from build123d import *

# Parameters (mm, degrees)
SKETCH1_R           = 2
BOSS_EXTRUDE1_DEPTH = 25
BOSS_EXTRUDE2_START = -25
SKETCH3_R           = 7
SKETCH3_R_2         = 2
BOSS_EXTRUDE2_DEPTH = 25
MOVE_FACE1_BY       = 2
MOVE_FACE1_2_BY     = 2
BOSS_EXTRUDE3_START = -25
BOSS_EXTRUDE3_DEPTH = 25


with BuildPart() as part:
    # Sketch1 → Boss-Extrude1 (new body)
    with BuildSketch(Plane(origin=(0, 0, 0), x_dir=(1, 0, 0), z_dir=(0, 1, 0))):
        with BuildLine():
            Line((-5, 0), (-5, 29.5))
            ThreePointArc((-5, 29.5), (0, 34.5), (5, 29.5))
            Line((5, 29.5), (5, 0))
            ThreePointArc((5, 0), (0, -5), (-5, 0))
        make_face()
        with Locations(Location((0, 29.5, 0), (0, 0, 270))):
            Circle(SKETCH1_R, mode=Mode.SUBTRACT)
        with Locations(Location((0, 0, 0), (0, 0, 270))):
            Circle(SKETCH1_R, mode=Mode.SUBTRACT)
    extrude(amount=BOSS_EXTRUDE1_DEPTH)

    # Sketch3 → Boss-Extrude2 (add)
    # profile 1 of 2: a face of its own
    with BuildSketch(Plane(origin=(0, 25, 0), x_dir=(1, 0, 0), z_dir=(0, 1, 0)).offset(BOSS_EXTRUDE2_START)):
        with Locations((0, 29.5)):
            Circle(SKETCH3_R)
        with Locations(Location((0, 29.5, 0), (0, 0, 270))):
            Circle(SKETCH3_R_2, mode=Mode.SUBTRACT)
    # profile 2 of 2: a face of its own
    with BuildSketch(Plane(origin=(0, 25, 0), x_dir=(1, 0, 0), z_dir=(0, 1, 0)).offset(BOSS_EXTRUDE2_START)):
        Circle(SKETCH3_R)
        with Locations(Location((0, 0, 0), (0, 0, 270))):
            Circle(SKETCH3_R_2, mode=Mode.SUBTRACT)
    extrude(amount=BOSS_EXTRUDE2_DEPTH)

    # Move Face1: a curved face moved inward by 2.0
    add(Solid.thicken(part.faces().sort_by_distance((0, 12.5, -31.5))[0], -MOVE_FACE1_BY), mode=Mode.SUBTRACT)

    # Move Face1 2: a curved face moved inward by 2.0
    add(Solid.thicken(part.faces().sort_by_distance((0, 12.5, -2))[0], -MOVE_FACE1_2_BY), mode=Mode.SUBTRACT)

    # Sketch5 → Boss-Extrude3 (add)
    with BuildSketch(Plane(origin=(0, 25, 0), x_dir=(1, 0, 0), z_dir=(0, 1, 0)).offset(BOSS_EXTRUDE3_START)):
        with BuildLine():
            Line((-2.6, 3.039736831), (-2.6, -3.039736831))
            ThreePointArc((-2.6, -3.039736831), (-4, 0), (-2.6, 3.039736831))
        make_face()
    extrude(amount=BOSS_EXTRUDE3_DEPTH)


solid = part.part
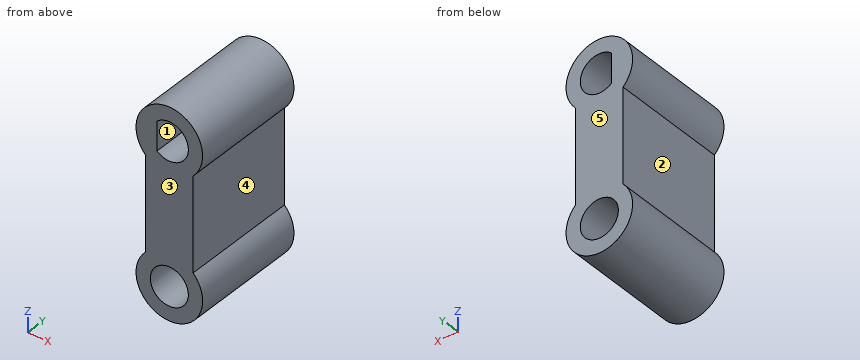
Verification items for the finished model (mm, model axes). Face numbers are marked on the shaded views. A direction names the side the tool comes from. Coordinates: 2 decimals unless noted, no trailing zeros. Write each loop counter-clockwise with the first axis right and the second up, starting at its lowest first coordinate (ties: lowest second). Pieces come first, ordered by that corner, then holes. Notation, with made-up numbers: (-15, 80.25) -> (27, 80.25) arc R23 ccw to (27, 118.25) -> close; hole circle Ø11 at (60, 11.25). An arc over 180 degrees is marked (long way). One line per item, written item: value. Start each with the question number.
Q1. Access from +Z, -Z, +X, -X, +Y, -Y to the whole of each face (thin tool, end or side, straight path). Record for the marked faces 1, 2 and 3.
Q2. Cross-section at D-D on z = 0. Enter the section's corners in (x, y).
Q3. Cross-section at A-A on x = 0. Enter the section's corners in (y, z), and give its area (4 significant figures).
Q4. Cross-section at B-B on z = -29.5. Enter the section's corners in (x, y), and give its area (3 significant figures).
Q5. Mould release check, pull along Z, two halves, no side actions. Record for the marked faces 4 and 5: pulls with the +Z half, pulls with the -Z half, needs draft (parallel to the pull), parting line crosses it, or undercut.
Q6. Cross-section at C-C on y = 17.75. Enter the section's corners in (x, z).
Q7. Go/stop test with flat-tipped pins: P1, Ø1, axis at y = 18.5, z = -10, coming from the +X side; P2, Ø12, axis at y = 8, z = -23, coming from the -X side. Record where each tip stops, or that it passes through.
Q8. Thickness scan on L1, parallel to X at y = 13.5, z = -29.5; L2, parallel to Z at x = 1, y = 19; L3, parallel to X at y = 17, z = -24. Record the ranges inside material, lowest first. Write a range as from..to.
Checked values:
1. face 1: +Y, -Y
1. face 2: -X, +Y, -Y
1. face 3: +Z, -Z, +X, -X, -Y
2. outline: (-7, 0) -> (-2.6, 0) -> (-2.6, 25) -> (-7, 25) -> close; (4, 0) -> (7, 0) -> (7, 25) -> (4, 25) -> close
3. outline: (0, -36.5) -> (25, -36.5) -> (25, -33.5) -> (0, -33.5) -> close; (0, -25.5) -> (25, -25.5) -> (25, -4) -> (0, -4) -> close; (0, 4) -> (25, 4) -> (25, 7) -> (0, 7) -> close
3. area: 687.5 mm²
4. outline: (-7, 0) -> (-4, 0) -> (-4, 25) -> (-7, 25) -> close; (4, 0) -> (7, 0) -> (7, 25) -> (4, 25) -> close
4. area: 150 mm²
5. face 4: undercut
5. face 5: needs draft
6. outline: (-5, -24.6) arc R7 ccw (long way) to (5, -24.6) -> (5, -4.9) arc R7 ccw (long way) to (-5, -4.9) -> close; hole circle Ø8 at (0, -29.5); hole (-2.6, -3.04) arc R4 ccw (long way) to (-2.6, 3.04) -> close
7. P1: stops at x = 5
7. P2: stops at x = -6.98
8. L1: x = -7..-4, 4..7
8. L2: z = -36.43..-33.37, -25.63..-3.87, 3.87..6.93
8. L3: x = -5..5
